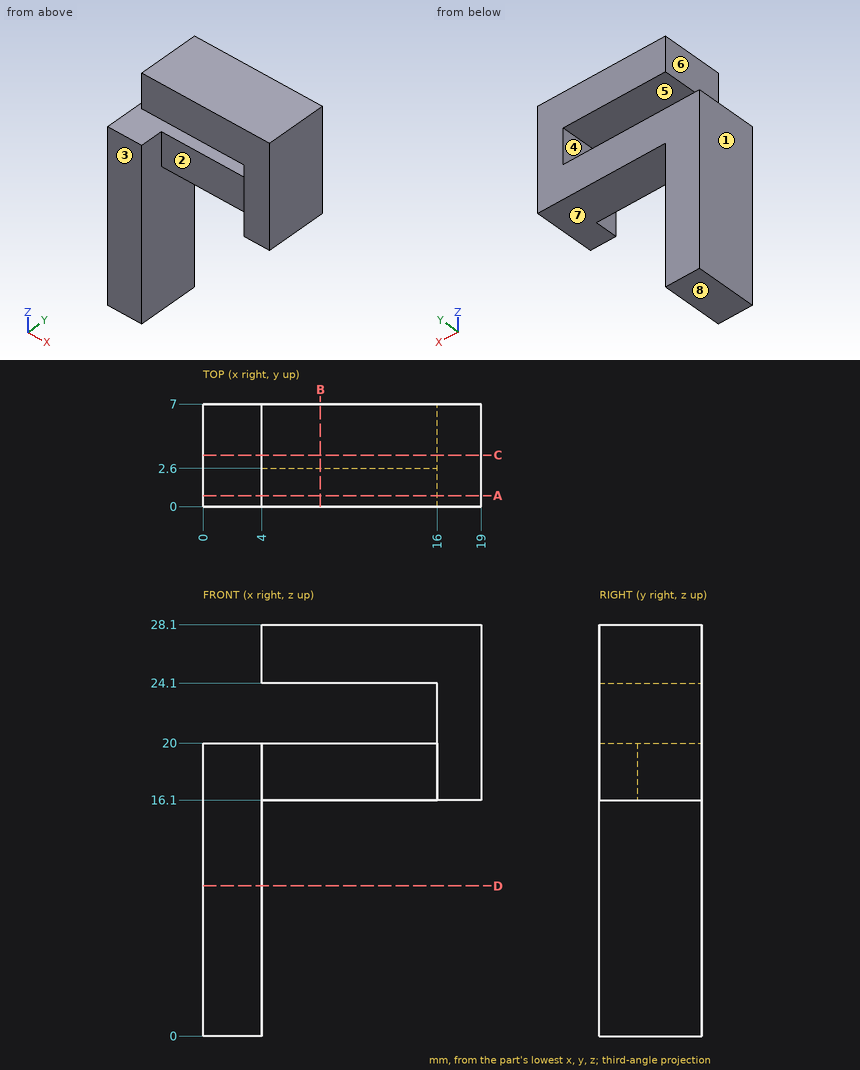
Part print with two shaded views. Sizes in mm from the minimum x, y, z corner. A direction names the side the tool comes from. Coordinates: 2 decimals unless noted, no trailing zeros. Loops run counter-clockwise (first coordinate to the right, second up) from the corner with the lowest first, then second, coordinate; pieces in that order, holes last. Notation, with made-up numbers: M 24,0.25 L 34,0.25 A21 cw 34,34.25 Z; hole C 47.25,-7.75 d10. An arc over 180 degrees is marked long. Use CSV: the item, a comma, the result in double quotes. Start each with the question number.
1. Band-saw the part on D-D, the plane z = 10.25. List the corners of the cut face in (x, y), then the cut area to 3 significant figures.
2. Probe probe 1 along Z at (x, y) = (14.75, 5.5); probe 2 along Z at (x, y) = (15, 2); probe 3 along X at (y, z) = (0.5, 24.5). List the from-to ranges inside material, lowest first. Write a range as [from, to].
3. Two-plate mould, pull along X, no slides. Class the marked faces 1, 2, 3 and 4: pulls with the +X half, pulls with the -X half, needs draft (parallel to the pull), parting line crosses it, or undercut.
4. Band-saw the part on C-C, the plane y = 3.5. List the corners of the cut face in (x, z), then the cut area to 3 significant figures.
5. Band-saw the part on A-A, the plane y = 0.75. List the corners of the cut face in (x, z).
6. Tool access for the marked faces 5, 6, 7 and 8: list every direction of +Z, -Z, +X, -X, +Y, -Y with a clear straight run to the whole face (end or side of a thin tool).
7. Band-saw the part on B-B, the plane x = 8. List the corners of the cut face in (y, z), then the cut area to 3 significant figures.
8. Flat gauge pins, fed straight in: pin 1 (3.5 mm diameter, centred on y = 4.5, z = 7, fed in from +X); pin 2 (2 mm diameter, centred on x = 13, y = 4.5, fed in from -Z); pin 3 (4.5 mm diameter, centred on x = 9.5, z = 19, fed in from -Y). Where does each tip first touch, or does it go through?
Entries:
1,outline,"M 0,0 L 4,0 L 4,7 L 0,7 Z"
1,area,"28.0 mm2"
2,probe 1,"z = [16.1, 20], [24.1, 28.1]"
2,probe 2,"z = [24.1, 28.1]"
2,probe 3,"x = [4, 19]"
3,face 1,"pulls with the -X half"
3,face 2,"undercut"
3,face 3,"needs draft"
3,face 4,"undercut"
4,outline,"M 0,0 L 4,0 L 4,16.1 L 19,16.1 L 19,28.1 L 4,28.1 L 4,24.1 L 16,24.1 L 16,20 L 0,20 Z"
4,area,"211 mm2"
5,outline,"M 0,0 L 4,0 L 4,20 L 0,20 Z; M 4,24.1 L 16,24.1 L 16,16.1 L 19,16.1 L 19,28.1 L 4,28.1 Z"
6,face 5,"-X, +Y, -Y"
6,face 6,"+Z, -X, +Y, -Y"
6,face 7,"-Z, +X, +Y, -Y"
6,face 8,"-Z, +X, -X, +Y, -Y"
7,outline,"M 0,24.1 L 7,24.1 L 7,28.1 L 0,28.1 Z; M 2.6,16.1 L 7,16.1 L 7,20 L 2.6,20 Z"
7,area,"45.2 mm2"
8,pin 1,"stops at x = 4"
8,pin 2,"stops at z = 16.1"
8,pin 3,"stops at y = 2.6"
